Can you work these out from the model? Positions are in its coordinate system, mm. A direction names the side the tool comes from. Coordinates: 2 decimals unless noted, no trailing zeros. Write each loop counter-clockwise with the first axis right and the second up, starting at its lowest first coordinate (ties: lowest second). Pieces come first, ordered by that corner, then holes. Notation, with made-up numbers: M 15,25.5 L 35,25.5 A33 ccw 35,64.5 Z; hole C -40,-33.75 d9. An arc over 180 degrees is marked long. Use one line per item in the form item = value. Start each with the question number.
```python
from build123d import *

# Parameters (mm, degrees)
PAD_DEPTH    = 56.05
SKETCH001_R  = 0.5
POCKET_DEPTH = 70
PAD001_DEPTH = 5


with BuildPart() as part:
    # Sketch → Pad (new body)
    with BuildSketch(Plane.XY):
        with BuildLine():
            Line((-5.067001, 3.25), (-1e-06, 3.25))
            ThreePointArc((-2e-06, -3.25), (3.253286, 0), (-1e-06, 3.25))
            Line((-2e-06, -3.25), (-5.067001, -3.25))
            Line((-5.067001, -3.25), (-5.067001, 3.25))
        make_face()
    extrude(amount=PAD_DEPTH)

    # Sketch001 (on Face6 of Pad) → Pocket (cut)
    with BuildSketch(Plane.XY.offset(56.05)):
        with Locations((-1.27, 0)):
            Circle(SKETCH001_R)
        with Locations((1.27, 0)):
            Circle(SKETCH001_R)
    extrude(amount=-POCKET_DEPTH, mode=Mode.SUBTRACT)

    # Sketch002 (on Face4 of Pocket) → Pad001 (join)
    with BuildSketch(Plane(origin=(0, 0, 0), x_dir=(1, 0, 0), z_dir=(0, 0, -1))):
        with BuildLine():
            Line((-3.84, 1.905), (-3.84, -1.905))
            ThreePointArc((-5.04, -1.879774), (-4.452472, -2.485689), (-3.84, -1.905))
            Line((-5.04, 1.879643), (-5.04, -1.879774))
            ThreePointArc((-3.84, 1.905), (-4.452379, 2.478133), (-5.04, 1.879643))
        make_face()
    extrude(amount=PAD001_DEPTH)


solid = part.part
```
1) Please list where these lines run through material, in increasing order: line 1 (Y direction, x = -1.27, z = 30.5); line 2 (Y direction, x = 1.27, z = 12); line 3 (Z direction, x = -2, y = -1.25).
2) Suppose I cut it at A-A on y = 0. State how many separate pieces and enclosed holes the cut face has, and give its area (3 significant figures).
3) Which directions (+Z, -Z, +X, -X, +Y, -Y) give clear straight access to the entire face, cutting with the end or side of a thin tool? Please do faces 1 (the face through (-3.84, 0, -2)), 2 (the face through (-4.44, -2.48, -2.46)), 3 (the face through (-5.067, 0, 28)).
4) If we mould it in two halves opening along Y, with no side actions, what happens to faces 4 (the face through (-2, -3.25, 28)), 5 (the face through (-5.04, 0, -2)), 6 (the face through (-0.808, -0.192, 28.417)), 7 (the face through (-3, 3.25, 28))? For each: +Y half, -Y half, draft (parallel to the pull), parting line (faces both ways), or undercut.
5) Will these pins go through, and if not, where does the flat tip stop? pin 1 Ø3 at (y, z) = (-0.5, -2.5) entering from +X; pin 2 Ø4 at (x, z) = (2, 41) entering from -Y; pin 3 Ø1.9 at (y, z) = (-0.5, -3.5) entering from -X.
6) Suppose I cut it at D-D on x = 1.27. Please give me the cut outline in (y, z).
7) Suppose I cut it at C-C on z = 17. Please give me the cut outline in (x, y).
8) Suppose I cut it at B-B on x = -1.27. Please give me the cut outline in (y, z).
Computed values:
q1.line_1 = -3.25 to -0.5, 0.5 to 3.25
q1.line_2 = -2.99 to -0.5, 0.5 to 2.99
q1.line_3 = 0 to 56.05
q2.separate_pieces = 3
q2.enclosed_holes = 0
q2.area = 360 mm²
q3.face_1 = -Z, +X, +Y, -Y
q3.face_2 = -Z, -Y
q3.face_3 = +Z, -Z, -X, +Y, -Y
q4.face_4 = -Y half
q4.face_5 = draft
q4.face_6 = undercut
q4.face_7 = +Y half
q5.pin_1 = -3.84
q5.pin_2 = -3.25
q5.pin_3 = -5.04
q6.outline = M -2.99,0 L -0.5,0 L -0.5,56.05 L -2.99,56.05 Z; M 0.5,0 L 2.99,0 L 2.99,56.05 L 0.5,56.05 Z
q7.outline = M -5.07,-3.25 L 0,-3.25 A3.25 ccw 0,3.25 L -5.07,3.25 Z; hole C -1.27,0 d1; hole C 1.27,0 d1
q8.outline = M -3.25,0 L -0.5,0 L -0.5,56.05 L -3.25,56.05 Z; M 0.5,0 L 3.25,0 L 3.25,56.05 L 0.5,56.05 Z
